Input: part model. Units: mm. Frame: model coordinates. A direction names the side the tool comes from. Give positions to 0.01 mm unless a question says otherwise; leave off trailing zeros. Loops run counter-clockwise (first coordinate to the right, second up) from the corner with the lowest first, then second, coordinate; pieces in that order, holes last. Notation, with made-up numbers: (34, 40.5) - (41, 40.5) arc R24 cw to (41, 77.5) - close; hole circle Ø6 at (62, -38.5). An arc over 180 degrees is marked (long way). Answer as a JSON object with one key per item and string values.
from build123d import *

# Parameters (mm, degrees)
BLOCK_START           = 543
BLOCK_1_DEPTH         = 12
BLOCK_EDGE_FILLET_1_R = 5
PIPE_1_PROFILE_R      = 5


with BuildPart() as part:
    # Block sketch 1 → Block 1 (new body)
    with BuildSketch(Plane.XY.offset(BLOCK_START)):
        with BuildLine():
            Line((683, -117), (832, -117))
            ThreePointArc((832, -117), (842.606601718, -112.606601718), (847, -102))
            Line((847, -102), (847, 102))
            ThreePointArc((847, 102), (842.606601718, 112.606601718), (832, 117))
            Line((832, 117), (683, 117))
            ThreePointArc((683, 117), (672.393398282, 112.606601718), (668, 102))
            Line((668, 102), (668, -102))
            ThreePointArc((668, -102), (672.393398282, -112.606601718), (683, -117))
        make_face()
    extrude(amount=BLOCK_1_DEPTH)

    # Block edge fillet 1
    block_edge_fillet_1_edges = [part.edges().sort_by_distance(p)[0] for p in [
        (847, 0, 543),
        (842.606601718, -112.606601718, 543),
        (757.5, -117, 543),
        (672.393398282, -112.606601718, 543),
        (842.606601718, -112.606601718, 555),
        (847, 0, 555),
        (842.606601718, 112.606601718, 555),
        (757.5, 117, 555),
        (672.393398282, 112.606601718, 555),
        (668, 0, 555),
        (672.393398282, -112.606601718, 555),
        (668, 0, 543),
        (757.5, -117, 555),
        (672.393398282, 112.606601718, 543),
        (757.5, 117, 543),
        (842.606601718, 112.606601718, 543),
    ]]
    fillet(block_edge_fillet_1_edges, radius=BLOCK_EDGE_FILLET_1_R)


with BuildPart() as body_2:
    # Pipe 1: sweep along a curve in space
    with BuildLine() as pipe_1_path:
        Line((717.5, -97, 555), (717.5, -97, 562.7))
        ThreePointArc((717.5, -97, 562.7), (719.345227279, -97, 567.154772721), (723.8, -97, 569))
        Line((723.8, -97, 569), (791.2, -97, 569))
        ThreePointArc((791.2, -97, 569), (795.654772721, -97, 567.154772721), (797.5, -97, 562.7))
        Line((797.5, -97, 562.7), (797.5, -97, 555))
    # Pipe 1 profile (on start of the path) → Pipe 1 (sweep)
    with BuildSketch(Plane(origin=(717.5, -97, 555), x_dir=(1, 0, 0), z_dir=(0, 0, 1))):
        Circle(PIPE_1_PROFILE_R)
    sweep(path=pipe_1_path.line)

    # Combine (weld / assembly of features): union part
    add(part.part)


solid = body_2.part
Item 1: Cut plane D-D (z = 558). Return loops of the section in (x, y).
Geometry check:
{"outline": "circle Ø10 at (717.5, -97); circle Ø10 at (797.5, -97)"}
Item 2: Access query for faces 4 (the face through (792.881, -98.915, 558.796)), 5 (the face through (669, -1, 553)). Directions: +Z, -Z, +X, -X, +Y, -Y. A direction counts if a zero-diameter tool reaches every point of the face in a straight line with its end or side. Return the directions, or none.
Geometry check:
{"face 4": "none", "face 5": "+Z, -X, +Y, -Y"}
Item 3: Cut plane B-B (x = 769.5). Return loops of the section in (y, z).
Geometry check:
{"outline": "(-117, 548) arc R5 ccw to (-112, 543) - (112, 543) arc R5 ccw to (117, 548) - (117, 550) arc R5 ccw to (112, 555) - (-112, 555) arc R5 ccw to (-117, 550) - close; circle Ø10 at (-97, 569)"}
Item 4: Mould query, pull axis Z, two halves, no side actions, for faces 1 (the face through (842.49, -112.72, 548.99)), 2 (the face through (756, 2, 543)), 3 (the face through (722.119, -98.915, 558.904)). Classes: released by +Z, released by -Z, zero draft, split by the parting line, or undercut.
Geometry check:
{"face 1": "zero draft", "face 2": "released by -Z", "face 3": "undercut"}
Item 5: Cut plane C-C (x = 695.5). Return loops of the section in (y, z), then the cut area to 3 significant figures.
Geometry check:
{"outline": "(-117, 548) arc R5 ccw to (-112, 543) - (112, 543) arc R5 ccw to (117, 548) - (117, 550) arc R5 ccw to (112, 555) - (-112, 555) arc R5 ccw to (-117, 550) - close", "area": "2,790 mm2"}
Item 6: Material intervals for line 1 (Y direction, x = 781, z = 568.5); line 2 (Z direction, x = 807, y = -42); line 3 (X direction, y = -95, z = 562.5), sorted ascending. Write a range as [from, to].
Geometry check:
{"line 1": "y = [-101.97, -92.03]", "line 2": "z = [543, 555]", "line 3": "x = [712.92, 722.08], [792.92, 802.08]"}
Item 7: Cut plane A-A (y = -97). Return loops of the section in (x, z).
Geometry check:
{"outline": "(668, 548) arc R5 ccw to (673, 543) - (842, 543) arc R5 ccw to (847, 548) - (847, 550) arc R5 ccw to (842, 555) - (802.5, 555) - (802.5, 562.7) arc R11.3 ccw to (791.2, 574) - (723.8, 574) arc R11.3 ccw to (712.5, 562.7) - (712.5, 555) - (673, 555) arc R5 ccw to (668, 550) - close; hole (722.5, 555) - (792.5, 555) - (792.5, 562.7) arc R1.3 ccw to (791.2, 564) - (723.8, 564) arc R1.3 ccw to (722.5, 562.7) - close"}
